Could you check a few things on this model? Use its own coordinates, in mm. Face numbers are marked on the shaded views. A direction names the side the tool comes from. Round coordinates to 2 decimals unless told otherwise and drop trailing zeros. Write each loop counter-clockwise with the first axis right and the second up, starting at its lowest first coordinate (ties: lowest second). Pieces come first, ordered by that corner, then holes. Notation, with made-up numbers: (-8, -36.75) - (35, -36.75) arc R16 ccw to (35, -28.75) - close; hole circle Ø11 at (64.25, 18.5). An arc over 180 degrees is marked (long way). Put each result on its own line as item: value.
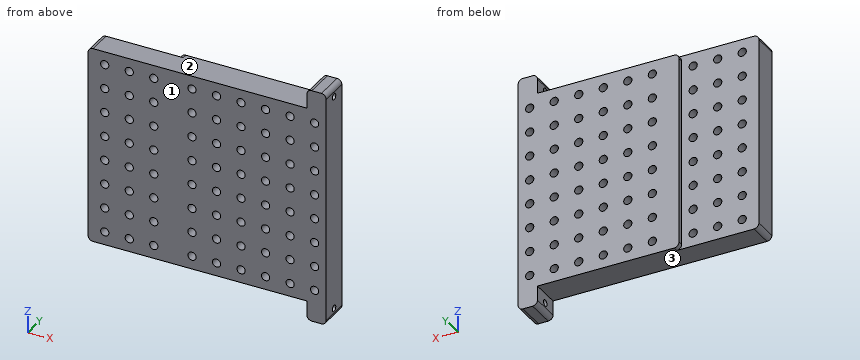
from build123d import *

# Parameters (mm, degrees)
BOSS_EXTRUDE1_DEPTH  = 205
M8_CLEARANCE_HOLE1_D = 8.5
FILLET1_R            = 5
SKETCH5_W            = 20
SKETCH5_H            = 30
BOSS_EXTRUDE2_DEPTH  = 20
SKETCH7_R            = 3.3
CUT_EXTRUDE1_DEPTH   = 20
FILLET2_R            = 5


with BuildPart() as part:
    # Sketch1 → Boss-Extrude1 (new body)
    with BuildSketch(Plane.XY):
        Polygon((-80, 0), (0, 0), (0, 5), (166.6, 5), (166.6, -25), (-80, -25), align=None)
    extrude(amount=BOSS_EXTRUDE1_DEPTH)

    # M8 Clearance Hole1 (through all)
    with Locations(Plane(origin=(0, 5, 0), x_dir=(1, 0, 0), z_dir=(0, 1, 0))):
        with Locations((-12, -13.6), (-62.8, -13.6), (-113.6, -13.6), (-62.8, -64.4), (-113.6, -64.4), (-62.8, -115.2), (-113.6, -115.2), (-62.8, -166), (-113.6, -166), (-12, -64.4), (-12, -115.2), (-12, -166), (53, -13.6), (103.8, -13.6), (154.6, -13.6), (103.8, -64.4), (154.6, -64.4), (103.8, -115.2), (154.6, -115.2), (103.8, -166), (154.6, -166), (53, -64.4), (53, -115.2), (53, -166), (-62.8, -39), (-12, -39), (53, -39), (103.8, -39), (154.6, -39), (154.6, -89.8), (103.8, -89.8), (53, -89.8), (-12, -89.8), (-62.8, -89.8), (-62.8, -140.6), (-12, -140.6), (53, -140.6), (103.8, -140.6), (154.6, -140.6), (154.6, -191.4), (103.8, -191.4), (53, -191.4), (-12, -191.4), (-62.8, -191.4), (-37.4, -13.6), (-37.4, -64.4), (-37.4, -115.2), (-37.4, -166), (-37.4, -191.4), (-37.4, -39), (-37.4, -89.8), (-37.4, -140.6), (129.2, -13.6), (129.2, -64.4), (129.2, -115.2), (129.2, -166), (129.2, -39), (129.2, -89.8), (129.2, -140.6), (129.2, -191.4), (78.4, -13.6), (78.4, -64.4), (78.4, -115.2), (78.4, -166), (78.4, -39), (78.4, -89.8), (78.4, -140.6), (78.4, -191.4), (27.6, -13.6), (27.6, -64.4), (27.6, -115.2), (27.6, -166), (27.6, -39), (27.6, -89.8), (27.6, -140.6), (27.6, -191.4)):
            Hole(M8_CLEARANCE_HOLE1_D / 2)

    # Fillet1
    fillet1_edges = [part.edges().sort_by_distance(p)[0] for p in [
        (0, 2.5, 205),
        (-80, -12.5, 205),
        (0, 2.5, 0),
        (-80, -12.5, 0),
    ]]
    fillet(fillet1_edges, radius=FILLET1_R)

    # Sketch5 → Boss-Extrude2 (add)
    with BuildSketch(Plane.XY.offset(205)):
        with Locations((156.6, -10)):
            Rectangle(SKETCH5_W, SKETCH5_H)
    boss_extrude2 = extrude(amount=BOSS_EXTRUDE2_DEPTH)

    # Sketch7 → Cut-Extrude1 (cut)
    with BuildSketch(Plane.ZY.offset(-146.6)):
        with Locations((215, -10)):
            Circle(SKETCH7_R)
    cut_extrude1 = extrude(amount=-CUT_EXTRUDE1_DEPTH, mode=Mode.SUBTRACT)

    # Mirror1: Boss-Extrude2, Cut-Extrude1 across plane
    add(boss_extrude2.mirror(Plane.XY.offset(102.5)))
    add(cut_extrude1.mirror(Plane.XY.offset(102.5)), mode=Mode.SUBTRACT)

    # Fillet2
    fillet2_edges = [part.edges().sort_by_distance(p)[0] for p in [
        (166.6, -10, 225),
        (146.6, -10, 225),
        (166.6, -10, -20),
        (146.6, -10, -20),
    ]]
    fillet(fillet2_edges, radius=FILLET2_R)


solid = part.part
(1) For the marked faces 1, 2 and 3, which set-ups out of +Z, -Z, +X, -X, +Y, -Y let a thin tool reach every point of the face, with its end or its side?
Values found:
face 1: +Z, -Z, +X, -X, -Y
face 2: +Z, -X, +Y, -Y
face 3: -Z, -X, +Y, -Y
(2) Imagine slicing it at C-C, the plane x = 95.5. List the corners of the cut face in (y, z) for me.
Values found:
outline: (-25, 0) - (5, 0) - (5, 205) - (-25, 205) - close
(3) I'm going to push flat-ended pins straight in: pin 1 (3 mm diameter, centred on x = -35, z = 58, fed in from +Y); pin 2 (10 mm diameter, centred on x = 83.5, y = -2.5, fed in from +Z); pin 3 (1.5 mm diameter, centred on x = -5, y = -15, fed in from -Z). Where does each tip first touch, or does it pass through?
Values found:
pin 1: stops at y = 0
pin 2: stops at z = 205
pin 3: stops at z = 0
(4) Please list where these lines run through material, in increasing order: probe 1 along Z at (x, y) = (70, -11); probe 2 along Y at (x, z) = (-60, 78); probe 3 along Z at (x, y) = (147, -22.25). Write a range as from..to.
Values found:
probe 1: z = 0..205
probe 2: y = -25..0
probe 3: z = -16.96..221.96
(5) Imagine slicing it at B-B, the plane x = -37.4. Give the number of separate pieces and of enclosed holes in the cut face, then the cut area to 4 significant figures.
Values found:
separate pieces: 9
enclosed holes: 0
area: 3,425 mm^2
(6) Imagine slicing it at A-A, the plane z = 77.5. List the corners of the cut face in (x, y) for me, then the cut area to 3 significant figures.
Values found:
outline: (-80, -25) - (166.6, -25) - (166.6, 5) - (0, 5) - (0, 0) - (-80, 0) - close
area: 7,000 mm^2
